from build123d import *

# Parameters (mm, degrees)
SKETCH_1_R      = 1.45
EXTRUDE_1_DEPTH = 2
FILLET_1_R      = 3


with BuildPart() as part:
    # 草图1 → 凸台-拉伸1 (new body)
    with BuildSketch(Plane(origin=(0, 0, 0), x_dir=(1, 0, 0), z_dir=(0, 1, 0))):
        Polygon((45, 15), (15, 45), (0, 45), (0, 15), (0, 0), (15, 0), (45, 0), align=None)
        with Locations(Location((29, 7.5, 0), (0, 0, 270))):
            Circle(SKETCH_1_R, mode=Mode.SUBTRACT)
        with Locations(Location((39, 7.5, 0), (0, 0, 270))):
            Circle(SKETCH_1_R, mode=Mode.SUBTRACT)
        with Locations(Location((7.5, 24, 0), (0, 0, 270))):
            Circle(SKETCH_1_R, mode=Mode.SUBTRACT)
        with Locations(Location((7.5, 34, 0), (0, 0, 270))):
            Circle(SKETCH_1_R, mode=Mode.SUBTRACT)
        Polygon((15, 15), (15, 39.343145751), (39.343145751, 15), align=None, mode=Mode.SUBTRACT)
    extrude(amount=EXTRUDE_1_DEPTH)

    # 圆角1
    fillet_1_edges = [part.edges().sort_by_distance(p)[0] for p in [
        (15, 1, -45),
        (45, 1, -15),
        (45, 1, 0),
        (0, 1, 0),
        (0, 1, -45),
        (15, 1, -39.343145751),
        (15, 1, -15),
        (39.343145751, 1, -15),
    ]]
    fillet(fillet_1_edges, radius=FILLET_1_R)


solid = part.part
The model under review builds one solid part; all positions refer to its coordinate system, in mm. A direction names the side the tool comes from. Round coordinates to 2 decimals unless told otherwise and drop trailing zeros. Order: outer loops, then holes, each group sorted by start corner. A loop starts at its lowest first (then second) coordinate and runs counter-clockwise, first axis right, second up. Notation, with made-up numbers: (73.5, 53.5) - (107.5, 53.5) arc R23 cw to (107.5, 62.5) - close; hole circle Ø7 at (-35, 67). An arc over 180 degrees is marked (long way). Use one line per item in the form item = value.
Q1. Add section C-C on x = 39. Give the boundary of the cut face in (y, z), then the cut area to 3 significant figures.
Response values:
outline = (0, -21) - (2, -21) - (2, -8.95) - (0, -8.95) - close; (0, -6.05) - (2, -6.05) - (2, 0) - (0, 0) - close
area = 36.2 mm^2
Q2. To check wall thickness, follow line 1 (X direction, y = 1.1, z = -7.5); line 2 (X direction, y = 0.4, z = -6.5); line 3 (Z direction, x = 28, y = 1.1). State the ranges of each line that lie inside material, in increasing order.
Response values:
line_1 = 0 to 27.55, 30.45 to 37.55, 40.45 to 45
line_2 = 0 to 27.95, 30.05 to 37.95, 40.05 to 45
line_3 = -32 to -26.34, -15 to -8.55, -6.45 to 0
Q3. Mouldability with a two-part tool opening along X and no side actions: class faces 1 (the flat face through (45, 1, -8)), 2 (the flat face through (0, 1, -23)), 3 (the cylindrical face through (6.945, 0.986, -22.661)) as pulls with the +X half, pulls with the -X half, needs draft (parallel to the pull), parting line crosses it, or undercut.
Response values:
face_1 = pulls with the +X half
face_2 = pulls with the -X half
face_3 = undercut
Q4. Add section A-A on x = 7.5. Give the boundary of the cut face in (y, z), then the cut area to 3 significant figures.
Response values:
outline = (0, -45) - (2, -45) - (2, -35.45) - (0, -35.45) - close; (0, -32.55) - (2, -32.55) - (2, -25.45) - (0, -25.45) - close; (0, -22.55) - (2, -22.55) - (2, 0) - (0, 0) - close
area = 78.4 mm^2
Q5. Clearance check with flat-ended pins moving along their axes: P1, Ø0.6, axis at x = 28.5, y = 0.5, coming from the -Z side; P2, Ø1, axis at x = 29, z = -22.5, coming from the +Y side; P3, Ø1, axis at y = 0.5, z = -30, coming from the +X side. State where each tip first meets the part, or that it passes through.
Response values:
P1 = -31.8
P2 = through
P3 = 30.5
Q6. Add section D-D on y = 0.8. Give the boundary of the cut face in (x, z).
Response values:
outline = (0, -42) arc R3 ccw to (3, -45) - (13.76, -45) arc R3 ccw to (15.88, -44.12) - (44.12, -15.88) arc R3 ccw to (45, -13.76) - (45, -3) arc R3 ccw to (42, 0) - (3, 0) arc R3 ccw to (0, -3) - close; hole circle Ø2.9 at (7.5, -34); hole circle Ø2.9 at (7.5, -24); hole (15, -32.1) arc R3 ccw to (20.12, -34.22) - (34.22, -20.12) arc R3 ccw to (32.1, -15) - (18, -15) arc R3 ccw to (15, -18) - close; hole circle Ø2.9 at (29, -7.5); hole circle Ø2.9 at (39, -7.5)
Q7. Tool access review of faces 4 (the cylindrical face through (16.9, 1.01, -34.89)), 5 (the flat face through (30, 1, -30)): name each direction out of +Z, -Z, +X, -X, +Y, -Y from which nothing blocks a thin tool from reaching the whole face with its end or side.
Response values:
face_4 = +Y, -Y
face_5 = -Z, +X, +Y, -Y
Q8. Add section B-B on z = -7.5. Give the boundary of the cut face in (x, y), then the cut area to 3 significant figures.
Response values:
outline = (0, 0) - (27.55, 0) - (27.55, 2) - (0, 2) - close; (30.45, 0) - (37.55, 0) - (37.55, 2) - (30.45, 2) - close; (40.45, 0) - (45, 0) - (45, 2) - (40.45, 2) - close
area = 78.4 mm^2
